The listing builds one solid part. Answer for the finished solid, in the listing's coordinates (mm). Face numbers are marked on the shaded views. Coordinates: 2 decimals unless noted, no trailing zeros. Order: outer loops, then holes, each group sorted by start corner. A loop starts at its lowest first (then second) coordinate and runs counter-clockwise, first axis right, second up. Notation, with made-up numbers: (-28.75, 6.5) -> (13.25, 6.5) arc R25 ccw to (13.25, 24.5) -> close; hole circle Ø4 at (-11, 47.5). An arc over 180 degrees is marked (long way). Write each question's results on one line, items separated by ' | '. Start each with the question number.
(1) The part is cut by section A-A, the plane x = 0. Give the vertices of the cut face in (y, z) (3 decimals), then the cut area to 3 significant figures.
(2) The part is cut by section C-C, the plane y = -1. Give the vertices of the cut face in (x, z).
(3) Determine the mould class of the marked faces 1, 2 and 3 for opening direction X: +X half, -X half, draft (parallel to the pull), parting line (faces both ways), or undercut.
(4) The part is cut by section B-B, the plane z = 0. Give the vertices of the cut face in (x, y) (3 decimals), then the cut area to 3 significant figures.
(5) Given pin 1 (4 mm diameter, centred on x = 10.5, y = -5, fed in from +Z); pin 2 (2 mm diameter, centred on x = 13, y = -12, fed in from -Z); pin 3 (8 mm diameter, centred on y = -5, z = -20, fed in from -X); pin 4 (6 mm diameter, centred on x = -26.5, z = 2, fed in from +Y), each flat-ended and moving along its own axis, determine where each tip first touches the part or whether it passes through.
(6) Straight lines are drawn through the part: L1, parallel to Z at x = 0, y = -11.65; L2, parallel to Y at x = -21, z = 14.5; L3, parallel to Y at x = 6, z = 9.5 (3 decimals). For each, find the intervals that lie inside material, in ascending order.
```python
from build123d import *

# Parameters (mm, degrees)
F0_R     = 38.1
F0_R_2   = 22.86
F1_DEPTH = 12.7
F2_R     = 3.048
F3_DEPTH = 9.525


with BuildPart() as f1:
    # F0 (on Front) → F1 (new body)
    with BuildSketch(Plane.XZ):
        Circle(F0_R)
        Circle(F0_R_2, mode=Mode.SUBTRACT)
    extrude(amount=F1_DEPTH)

    # F2
    f2_edges = [f1.edges().sort_by_distance(p)[0] for p in [
        (-38.1, -12.7, 0),
    ]]
    fillet(f2_edges, radius=F2_R)

    # F0 (on Front) → F3 (join)
    with BuildSketch(Plane.XZ):
        Circle(F0_R_2)
    extrude(amount=F3_DEPTH)

    # F4 (on face) → F5 (revolve)
    with BuildSketch(Plane.XZ.offset(12.7)):
        with BuildLine():
            Line((-25.076632, 11.43), (-25.076632, 17.526))
            ThreePointArc((-25.076632, 17.526), (-28.124632, 14.478), (-25.076632, 11.43))
        make_face()
        with BuildLine():
            Line((-25.076632, -17.526), (-25.076632, -11.43))
            ThreePointArc((-25.076632, -11.43), (-28.124632, -14.478), (-25.076632, -17.526))
        make_face()
    revolve(axis=Axis((-25.076632, -12.7, -0.637533), (0, 0, -1)))

    # F4 (on face) → F6 (revolve)
    with BuildSketch(Plane.XZ.offset(12.7)):
        with BuildLine():
            Line((0, 25.908), (0, 32.004))
            ThreePointArc((0, 32.004), (-3.048, 28.956), (0, 25.908))
        make_face()
        with BuildLine():
            Line((0, -32.004), (0, -25.908))
            ThreePointArc((0, -25.908), (-3.048, -28.956), (0, -32.004))
        make_face()
    revolve(axis=Axis((0, -12.7, 0.300789), (0, 0, -1)))

    # F4 (on face) → F7 (revolve)
    with BuildSketch(Plane.XZ.offset(12.7)):
        with BuildLine():
            Line((25.076632, 11.43), (25.076632, 17.526))
            ThreePointArc((25.076632, 17.526), (22.028632, 14.478), (25.076632, 11.43))
        make_face()
        with BuildLine():
            Line((25.076632, -17.526), (25.076632, -11.43))
            ThreePointArc((25.076632, -11.43), (22.028632, -14.478), (25.076632, -17.526))
        make_face()
    revolve(axis=Axis((25.076632, -12.7, 0.300787), (0, 0, -1)))


solid = f1.part
```
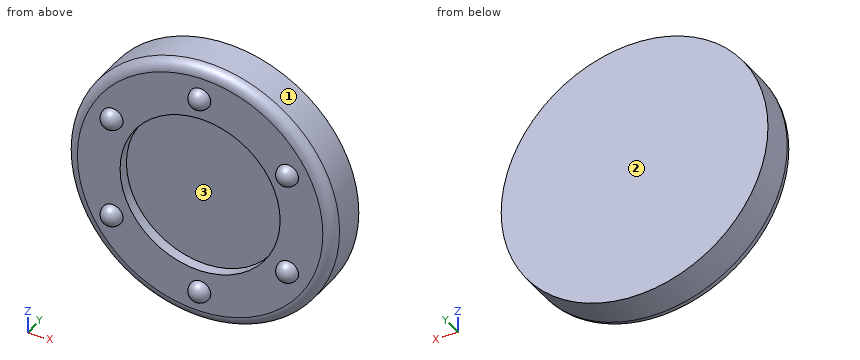
Established:
1) outline: (-12.7, -35.052) arc R3.048 ccw to (-9.652, -38.1) -> (0, -38.1) -> (0, 38.1) -> (-9.652, 38.1) arc R3.048 ccw to (-12.7, 35.052) -> (-12.7, 32.004) arc R3.048 ccw to (-12.7, 25.908) -> (-12.7, 22.86) -> (-9.525, 22.86) -> (-9.525, -22.86) -> (-12.7, -22.86) -> (-12.7, -25.908) arc R3.048 ccw to (-12.7, -32.004) -> close | area: 848 mm^2
2) outline: circle Ø76.2 at (0, 0)
3) face 1: parting line | face 2: draft | face 3: undercut
4) outline: (-38.1, -9.652) arc R3.048 ccw to (-35.052, -12.7) -> (-22.86, -12.7) -> (-22.86, -9.525) -> (22.86, -9.525) -> (22.86, -12.7) -> (35.052, -12.7) arc R3.048 ccw to (38.1, -9.652) -> (38.1, 0) -> (-38.1, 0) -> close | area: 819 mm^2
5) pin 1: stops at z = 37.14 | pin 2: stops at z = -35.58 | pin 3: stops at x = -34.58 | pin 4: stops at y = 0
6) L1: z = -37.35 to -22.86, 22.86 to 37.35 | L2: y = -12.7 to 0 | L3: y = -9.525 to 0
